Check sheet for the modelled part. Datum: model origin and axes. Units: mm. Face numbers are marked on the shaded views. A direction names the side the tool comes from. Round coordinates to 2 decimals unless told otherwise and drop trailing zeros. Loops run counter-clockwise (first coordinate to the right, second up) from the corner with the lowest first, then second, coordinate; pieces in that order, holes last. Notation, with made-up numbers: (34, -2) - (92, -2) arc R15 cw to (92, 24) - close; hole circle Ø1 at (-17.75, 13.25). An arc over 180 degrees is marked (long way). Put each result on its own line as item: value.
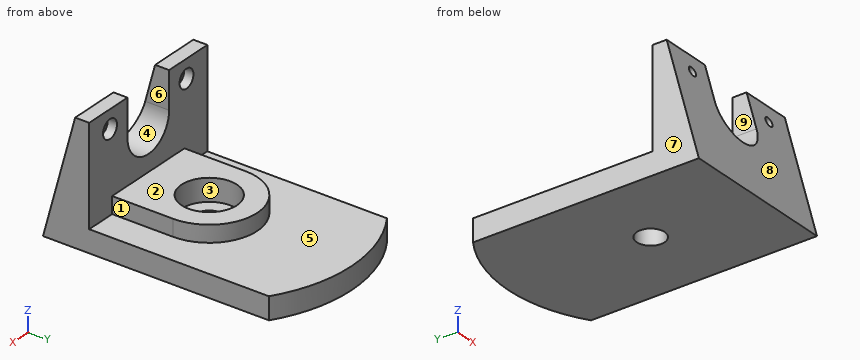
```python
from build123d import *

# Parameters (mm, degrees)
BOSS_EXTRUDE1_DEPTH                      = 42.5
CUT_EXTRUDE1_DEPTH                       = 54
CUT_EXTRUDE1_DEPTH_BACK                  = 13
BOSS_EXTRUDE2_DEPTH                      = 9
CBORE_FOR_M10_HEX_HEAD_BOLT1_D           = 15
CBORE_FOR_M10_HEX_HEAD_BOLT1_CBORE_D     = 30
CBORE_FOR_M10_HEX_HEAD_BOLT1_CBORE_DEPTH = 12
CUT_EXTRUDE2_DEPTH                       = 111
CUT_EXTRUDE2_DEPTH_BACK                  = 26
CBORE_FOR_M10_HEX_HEAD_BOLT2_D           = 5
CBORE_FOR_M10_HEX_HEAD_BOLT2_CBORE_D     = 10
CBORE_FOR_M10_HEX_HEAD_BOLT2_CBORE_DEPTH = 5


with BuildPart() as part:
    # Sketch1 → Boss-Extrude1 (new body, symmetric)
    with BuildSketch(Plane.YZ):
        Polygon((0, 0), (17.416697508, 65), (25, 65), (25, 12), (135, 12), (135, 0), align=None)
    extrude(amount=BOSS_EXTRUDE1_DEPTH, both=True)

    # Sketch3 → Cut-Extrude1 (cut, two sides)
    with BuildSketch(Plane.XY.offset(12)) as cut_extrude1_sk:
        with BuildLine():
            Line((-299.10474982, -47.63923197), (-42.5, 122.208644278))
            ThreePointArc((-42.5, 122.208644278), (0, 135), (42.5, 122.208644278))
            Line((42.5, 122.208644278), (299.10474982, -47.63923197))
            Line((299.10474982, -47.63923197), (299.10474982, 567.80954314))
            Line((299.10474982, 567.80954314), (-299.10474982, 567.80954314))
            Line((-299.10474982, 567.80954314), (-299.10474982, -47.63923197))
        make_face()
    extrude(amount=CUT_EXTRUDE1_DEPTH, mode=Mode.SUBTRACT)
    extrude(cut_extrude1_sk.sketch, amount=-CUT_EXTRUDE1_DEPTH_BACK, mode=Mode.SUBTRACT)

    # Sketch4 → Boss-Extrude2 (add)
    with BuildSketch(Plane.XY.offset(12)):
        with BuildLine():
            Line((-26, 25), (-26, 58))
            ThreePointArc((-26, 58), (0, 84), (26, 58))
            Line((26, 58), (26, 25))
            Line((26, 25), (-26, 25))
        make_face()
    extrude(amount=BOSS_EXTRUDE2_DEPTH)

    # CBORE for M10 Hex Head Bolt1 (through all)
    with Locations(Plane(origin=(0, 58, 21), x_dir=(1, 0, 0), z_dir=(0, 0, 1))):
        with Locations((0, 0)):
            CounterBoreHole(CBORE_FOR_M10_HEX_HEAD_BOLT1_D / 2, CBORE_FOR_M10_HEX_HEAD_BOLT1_CBORE_D / 2, CBORE_FOR_M10_HEX_HEAD_BOLT1_CBORE_DEPTH)

    # Sketch8 → Cut-Extrude2 (cut, two sides)
    with BuildSketch(Plane(origin=(0, 25, 0), x_dir=(-1, 0, 0), z_dir=(0, 1, 0))) as cut_extrude2_sk:
        with BuildLine():
            Line((-15, 65), (-15, 45))
            ThreePointArc((-15, 45), (0, 30), (15, 45))
            Line((15, 45), (15, 65))
            Line((15, 65), (-15, 65))
        make_face()
    extrude(amount=CUT_EXTRUDE2_DEPTH, mode=Mode.SUBTRACT)
    extrude(cut_extrude2_sk.sketch, amount=-CUT_EXTRUDE2_DEPTH_BACK, mode=Mode.SUBTRACT)

    # CBORE for M10 Hex Head Bolt2 (through all)
    with Locations(Plane(origin=(0, 25, 0), x_dir=(-1, 0, 0), z_dir=(0, 1, 0))):
        with Locations((0, 60), (27.5, 55), (0.084967263, 59.81697493), (-27.529393087, 55.058808224)):
            CounterBoreHole(CBORE_FOR_M10_HEX_HEAD_BOLT2_D / 2, CBORE_FOR_M10_HEX_HEAD_BOLT2_CBORE_D / 2, CBORE_FOR_M10_HEX_HEAD_BOLT2_CBORE_DEPTH)


solid = part.part
```
Item 1: Section check D-D on y = 105. Enter the section's corners in (x, z), then the cut area to 3 significant figures.
Filled sheet:
outline: (-42.5, 0) - (42.5, 0) - (42.5, 12) - (-42.5, 12) - close
area: 1,020 mm²
Item 2: Go/stop test with flat-tipped pins: pin 1 (12 mm diameter, centred on x = 0, y = 58, fed in from -Z); pin 2 (6.5 mm diameter, centred on x = -27.5, z = 55, fed in from -Y); pin 3 (6 mm diameter, centred on x = 27.53, z = 55.06, fed in from +Y); pin 4 (8 mm diameter, centred on x = -28.5, z = 57, fed in from +Y). Record where each tip stops, or that it passes through.
Filled sheet:
pin 1: through
pin 2: y = 13.87
pin 3: y = 20
pin 4: y = 25
Item 3: Section check C-C on z = 10.5. Enter the section's corners in (x, y), then the cut area to 3 significant figures.
Filled sheet:
outline: (-42.5, 2.81) - (42.5, 2.81) - (42.5, 122.21) arc R77 ccw to (-42.5, 122.21) - close; hole circle Ø30 at (0, 58)
area: 10,200 mm²
Item 4: Section check B-B on y = 53. Enter the section's corners in (x, z), then the cut area to 3 significant figures.
Filled sheet:
outline: (-42.5, 0) - (-5.59, 0) - (-5.59, 9) - (-14.14, 9) - (-14.14, 21) - (-26, 21) - (-26, 12) - (-42.5, 12) - close; (5.59, 0) - (42.5, 0) - (42.5, 12) - (26, 12) - (26, 21) - (14.14, 21) - (14.14, 9) - (5.59, 9) - close
area: 1,050 mm²
Item 5: Tool access check on the marked faces 1, 2, 3, 4 and 5. Record the directions out of +Z, -Z, +X, -X, +Y, -Y that give a thin tool (end or side, any length) a straight path to the whole face; none if there is none.
Filled sheet:
face 1: +Z, +X, +Y
face 2: +Z, +X, -X, +Y
face 3: +Z
face 4: +Z, +Y, -Y
face 5: +Z, +Y
Item 6: Thickness scan on line 1 (Z direction, x = -27, y = 22); line 2 (Z direction, x = -32.5, y = 100.5); line 3 (X direction, y = 38, z = 15.5). Record the ranges inside material, lowest first. Write a range as from..to.
Filled sheet:
line 1: 0..50.03, 59.97..65
line 2: 0..12
line 3: -26..26
Item 7: Release check for a two-part mould opening along X. For the marked faces 6, 7, 8 and 9 record: +X half, -X half, draft (parallel to the pull), parting line (faces both ways), or undercut.
Filled sheet:
face 6: undercut
face 7: -X half
face 8: draft
face 9: undercut
Item 8: Section check A-A on x = 0. Enter the section's corners in (y, z), then the cut area to 3 significant figures.
Filled sheet:
outline: (0, 0) - (50.5, 0) - (50.5, 9) - (43, 9) - (43, 21) - (25, 21) - (25, 30) - (8.04, 30) - close; (65.5, 0) - (135, 0) - (135, 12) - (84, 12) - (84, 21) - (73, 21) - (73, 9) - (65.5, 9) - close
area: 1,990 mm²
